Check sheet for the modelled part. Datum: model origin and axes. Units: mm. Face numbers are marked on the shaded views. A direction names the side the tool comes from. Coordinates: 2 decimals unless noted, no trailing zeros. Loops run counter-clockwise (first coordinate to the right, second up) from the corner with the lowest first, then second, coordinate; pieces in that order, holes last.
Autodesk Inventor part; units mm, degrees
ref_plane "Start plane" through (0, 0, 0) normal (0, 0, 1) x (1, 0, 0)
ref_plane "End plane" through (0, 0, 107.9074) normal (0, 0, 1) x (1, 0, 0)
ref_plane "YZ Plane" through (0, 0, 0) normal (1, 0, 0) x (0, 1, 0)
ref_plane "Start plane" through (0, 0, 0) normal (0, 0, 1) x (1, 0, 0)
ref_plane "End plane" through (0, 0, 107.9074) normal (0, 0, 1) x (1, 0, 0)
sketch "Sketch" plane through (0, 0, 0) normal (0, 0, 1) x (1, 0, 0)
  line L0 (0, 0) -> (0, 30)
  line L1 (0, 30) -> (30, 30)
  line L2 (30, 30) -> (30, 27.9696)
  line L3 (27.2392, 24.9791) -> (11.5215, 23.7217)
  line L4 (6, 17.7408) -> (6, 0)
  line L5 (6, 0) -> (0, 0) construction
  line L6 (15, 30) -> (15, 24) construction
  line L7 (30, 25.2) -> (30, 24) construction
  line L8 (30, 24) -> (15, 24) construction
  line L9 (0, 15) -> (0, -27) construction
  line L10 (-5.539, 0) -> (16.0067, 0) construction
  line L11 (0, 0) -> (0, -30)
  line L12 (0, -30) -> (30, -30)
  line L13 (30, -30) -> (30, -27.9696)
  line L14 (27.2392, -24.9791) -> (11.5215, -23.7217)
  line L15 (6, -17.7408) -> (6, 0)
  arc A0 (11.5215, 23.7217) -> (6, 17.7408) centre (12, 17.7408) ccw
  arc A1 (6, -17.7408) -> (11.5215, -23.7217) centre (12, -17.7408) ccw
  arc A2 (27.2392, 24.9791) -> (30, 27.9696) centre (27, 27.9696) ccw
  arc A3 (30, -27.9696) -> (27.2392, -24.9791) centre (27, -27.9696) ccw
  line L16 (0, 42) -> (0, -42) construction
  line L17 (-12.7637, 0) -> (37.8094, 0) construction
  point P0 (6, 23.28)
  point P1 (30, -25.2)
  point P2 (6, -23.28)
  point P3 (15, -30)
  point P4 (15, -24)
  dimension "d0" = 6
  dimension "d1" = 30
  dimension "d2" = 30
  dimension "d3" = 6
  dimension "d4" = 15
  dimension "d5" = 1.2
  dimension "d23" = 6
  dimension "d24" = 3
  dimension "d25" = 0
extrude "Body" add sketch "Sketch" along normal up to surface (107.9074 mm away) from surface at 0
sketch "Sketch3" plane through (0, 0, 0) normal (0, 0, 1) x (1, 0, 0)
  line L0 (0, 0) -> (10, 0)
ref_plane "Work Plane3" through (0, 0, 0) normal (0, -1, 0) x (1, 0, 0)
sketch "Sketch4" plane through (0, 0, 0) normal (0, -1, 0) x (1, 0, 0)
  line L0 (-2, 0) -> (12, 0)
  line L1 (-2, 107.9074) -> (12, 107.9074)
  dimension "d29" = 107.9074
sketch "Sketch5" plane through (0, 30, 107.9074) normal (0, 0, 1) x (1, 0, 0)
  line L0 (0, -30) -> (68.087, -30)
  circle A0 centre (31, -30) radius 25
  line L1 (31, -30) -> (31, 0.1301)
  line L2 (0, -60) -> (0, 0)
  line L3 (6, -12.2592) -> (6, -47.7408)
  arc A1 (27.2392, -5.0209) -> (30, -2.0304) centre (27, -2.0304) ccw
  line L4 (-62.4974, -26.9061) -> (-61.0279, -26.9061)
  line L5 (27.2392, -5.0209) -> (27.2392, 0)
  line L6 (0, 0) -> (30, 0)
  line L7 (27.2392, -5.0209) -> (11.5215, -6.2783)
  point P0 (-64.1158, -8.8185)
  point P1 (-63.0266, -8.8185)
  dimension "d30" = 50
  dimension "d32" = 6
  dimension "d33" = 27.9696
  dimension "d34" = 3
  dimension "d35" = 1.4696
  dimension "d36" = 3.7608
  dimension "d37" = 1.0892
  dimension "d38" = 30
  dimension "d39" = 31
  dimension "d41" = 5.0209
equation "\"d0\" = G_T"
equation "\"d1\" = 0.5 * G_H"
equation "\"d2\" = G_W"
equation "\"d3\" = G_T1"
equation "\"d4\" = G_C"
equation "\"d23\" = G_IR"
equation "\"d24\" = G_ER"
equation "\"d6\" = G_L"
equation "\"G_W\" = 30"
equation "\"G_H\" = 60"
equation "\"G_T\" = 6"
equation "\"G_T1\" = 6"
equation "\"G_NG\" = 0.08"
equation "\"G_ER\" = 3"
equation "\"G_IR\" = 6"
equation "\"G_C\" = 15"
equation "\"G_L\" = d29"
equation "\"ex\" = 0"
equation "\"G_OFFSET_START\" = 0"
equation "\"G_OFFSET_END\" = 0"
equation "\"d27\" = G_OFFSET_END + B_L"
equation "\"B_L\" = 107.90737"
properties part number "DIN1026-1 - U 60 - 107.907" material "Steel, Mild"
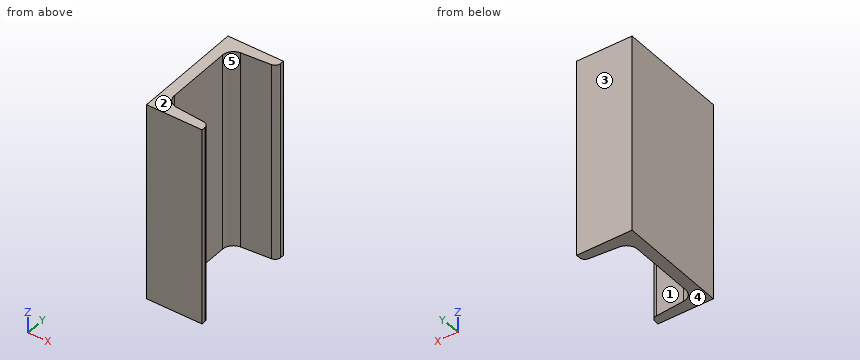
1) Section check D-D on y = 19.5. Enter the section's corners in (x, z), plus the area to 3 significant figures.
Answer sheet:
outline: (0, 0) - (6.26, 0) - (6.26, 107.91) - (0, 107.91) - close
area: 676 mm2
2) Section check A-A on x = 22.5. Enter the section's corners in (y, z), plus the area to 3 significant figures.
Answer sheet:
outline: (-30, 0) - (-24.6, 0) - (-24.6, 107.91) - (-30, 107.91) - close; (24.6, 0) - (30, 0) - (30, 107.91) - (24.6, 107.91) - close
area: 1,170 mm2
3) Section check B-B on z = 15. Enter the section's corners in (x, y), plus the area to 3 significant figures.
Answer sheet:
outline: (0, -30) - (30, -30) - (30, -27.97) arc R3 ccw to (27.24, -24.98) - (11.52, -23.72) arc R6 cw to (6, -17.74) - (6, 17.74) arc R6 cw to (11.52, 23.72) - (27.24, 24.98) arc R3 ccw to (30, 27.97) - (30, 30) - (0, 30) - close
area: 646 mm2
4) Scan lines: line 1 (Y direction, x = 21.5, z = 84); line 2 (Y direction, x = 14.5, z = 28); line 3 (X direction, y = -1.5, z = 85). Record each from-to range of solid material in increasing order.
Answer sheet:
line 1: y = -30 to -24.52, 24.52 to 30
line 2: y = -30 to -23.96, 23.96 to 30
line 3: x = 0 to 6
5) Set-up check for the marked faces 1 and 2: record each of +Z, -Z, +X, -X, +Y, -Y from which the full face is reachable in a straight line by a thin tool's end or side.
Answer sheet:
face 1: +Z, -Z, +X
face 2: +Z, +X, -X, +Y, -Y
6) Mould release check, pull along Y, two halves, no side actions. Record for the marked faces 3, 4 and 5: +Y half, -Y half, draft (parallel to the pull), parting line (faces both ways), or undercut.
Answer sheet:
face 3: +Y half
face 4: draft
face 5: undercut
7) Depth check by flat-ended pin: pin 1 (1.5 mm diameter, centred on y = 12.5, z = 30.5, fed in from +X); pin 2 (8 mm diameter, centred on y = -16, z = 79, fed in from +X). Enter the tip coordinate at first touch or a pass-through.
Answer sheet:
pin 1: stops at x = 6
pin 2: stops at x = 6.44
8) Section check C-C on y = 9.5. Enter the section's corners in (x, z), plus the area to 3 significant figures.
Answer sheet:
outline: (0, 0) - (6, 0) - (6, 107.91) - (0, 107.91) - close
area: 647 mm2
